For this review, take the finished solid that the model builds, in its own axes (mm). Give positions to 0.01 mm unless a question says otherwise; leave off trailing zeros. Write each loop counter-clockwise with the first axis right and the second up, starting at its lowest first coordinate (ties: lowest second). Pieces come first, ordered by that corner, then holes. Notation, with made-up numbers: (60, 22) -> (102, 22) arc R5 ccw to (102, 30) -> close; hole circle Ø7 at (-33, 75.25). An arc over 180 degrees is marked (long way). Write item = value, one per line.
```python
from build123d import *

# Parameters (mm, degrees)
BASPROSKE_W         = 16
BASPROSKE_H         = 6.8
TOOTHCUT_DEPTH      = 19.667619023
TEETHCUTS_COUNT     = 15
TEETHCUTS_ANGLE     = 336
BORSKE_R            = 2
BORE_DEPTH          = 50.000508
BOSS_EXTRUDE1_DEPTH = 16
CUT_EXTRUDE1_DEPTH  = 19.662017839


with BuildPart() as part:
    # BasProSke → Base-Revolve (revolve)
    with BuildSketch(Plane(origin=(0, 0, 0), x_dir=(1, 0, 0), z_dir=(0, 1, 0)), mode=Mode.PRIVATE) as base_revolve_sk:
        with Locations((8, 3.4)):
            Rectangle(BASPROSKE_W, BASPROSKE_H)
    revolve(base_revolve_sk.sketch.rotate(Axis((-10, 0, 0), (1, 0, 0)), 180), axis=Axis((-10, 0, 0), (1, 0, 0)))

    # TooCutSke → ToothCut (cut, through all)
    with BuildSketch(Plane(origin=(0, 0, 0), x_dir=(0, 0, -1), z_dir=(1, 0, 0))):
        with BuildLine():
            ThreePointArc((0.495059869, 4.974426271), (0, 4.999), (-0.495059869, 4.974426271))
            ThreePointArc((-0.495059869, 4.974426271), (-0.662158854, 5.91840511), (-1.185392978, 6.72167603))
            ThreePointArc((-1.185392978, 6.72167603), (0, 6.8254), (1.185392978, 6.72167603))
            ThreePointArc((1.185392978, 6.72167603), (0.662158854, 5.91840511), (0.495059869, 4.974426271))
        make_face()
    toothcut = extrude(amount=TOOTHCUT_DEPTH, mode=Mode.SUBTRACT)

    # TeethCuts: ToothCut ×15 about axis
    teethcuts_axis = Axis((-10, 0, 0), (1, 0, 0))
    for i in range(1, TEETHCUTS_COUNT):
        add(toothcut.rotate(teethcuts_axis, i * TEETHCUTS_ANGLE / (TEETHCUTS_COUNT - 1)), mode=Mode.SUBTRACT)

    # BorSke → Bore (cut, symmetric)
    with BuildSketch(Plane(origin=(0, 0, 0), x_dir=(0, 0, -1), z_dir=(1, 0, 0))):
        with Locations(Location((0, 0, 0), (0, 0, 180))):
            Circle(BORSKE_R)
    extrude(amount=BORE_DEPTH, both=True, mode=Mode.SUBTRACT)

    # Sketch1 → Boss-Extrude1 (add, through all)
    with BuildSketch(Plane(origin=(16, 0, 0), x_dir=(0, 0, -1), z_dir=(1, 0, 0))):
        with BuildLine():
            Line((-0.871779789, 1.8), (0.871779789, 1.8))
            ThreePointArc((0.871779789, 1.8), (0, 2), (-0.871779789, 1.8))
        make_face()
    extrude(amount=-BOSS_EXTRUDE1_DEPTH)

    # Sketch1<3> → Cut-Extrude1 (cut, through all)
    with BuildSketch(Plane(origin=(16, 0, 0), x_dir=(0, 0, -1), z_dir=(1, 0, 0))):
        with BuildLine():
            ThreePointArc((2.5, 0), (2.300797459, 0.977921803), (1.734935157, 1.8))
            Line((1.734935157, 1.8), (-1.734935157, 1.8))
            ThreePointArc((-1.734935157, 1.8), (-0.977921803, -2.300797459), (2.5, 0))
        make_face()
    extrude(amount=-CUT_EXTRUDE1_DEPTH, mode=Mode.SUBTRACT)


solid = part.part
```
(1) For pin 1 (3 mm diameter, centred on x = 12, y = 1, fed in from +Z); pin 2 (5 mm diameter, centred on x = 12, z = -1.5, fed in from +Y), all flat-tipped, find the tip position at first contact; note any pin that passes through.
Answers below:
pin_1 = 6.78
pin_2 = 6.7
(2) Take a section at C-C (z = 2.25). Write out the cut boundary in (x, y).
Answers below:
outline = (0, -6.09) -> (16, -6.09) -> (16, -1.09) -> (0, -1.09) -> close; (0, 1.09) -> (16, 1.09) -> (16, 4.46) -> (0, 4.46) -> close
(3) Take a section at A-A (z = 0). Write out the cut boundary in (x, y).
Answers below:
outline = (0, -6.8) -> (16, -6.8) -> (16, -2.5) -> (0, -2.5) -> close; (0, 1.8) -> (16, 1.8) -> (16, 5) -> (0, 5) -> close
(4) To check wall thickness, follow probe 1 along Y at (x, z) = (9, 5.5); probe 2 along Y at (x, z) = (9.5, 0); probe 3 along Z at (x, y) = (5, 3.25). State the ranges of each line that lie inside material, in increasing order.
Answers below:
probe_1 = -2.39 to -1.14, -0.04 to 1.2, 2.52 to 3.61
probe_2 = -6.8 to -2.5, 1.8 to 5
probe_3 = -5.97 to -4.4, -3.8 to 3.8, 4.4 to 5.97
(5) Take a section at B-B (z = 5.5). Write out the cut boundary in (x, y), plus the area to 3 significant figures.
Answers below:
outline = (0, -2.39) -> (16, -2.39) -> (16, -1.14) -> (0, -1.14) -> close; (0, -0.04) -> (16, -0.04) -> (16, 1.2) -> (0, 1.2) -> close; (0, 2.52) -> (16, 2.52) -> (16, 3.61) -> (0, 3.61) -> close
area = 57.2 mm^2
